The model under review builds one solid part; all positions refer to its coordinate system, in mm. A direction names the side the tool comes from. Round coordinates to 2 decimals unless told otherwise and drop trailing zeros. Loops run counter-clockwise (first coordinate to the right, second up) from the corner with the lowest first, then second, coordinate; pieces in that order, holes last. Notation, with made-up numbers: M 80.5,-28 L 85.5,-28 A18 ccw 85.5,-15 Z; hole C 70,-15.75 d8. An arc over 180 degrees is marked long. Use a Markdown table: item, result. Add a question column.
```python
from build123d import *

# Parameters (mm, degrees)
BOX_W           = 36
BOX_H           = 36
BOX_DEPTH       = 36
SKETCH_R        = 3.5
POCKET_DEPTH    = 36.001
SKETCH004_R     = 7
POCKET001_DEPTH = 13
SKETCH001_R     = 7
POCKET002_DEPTH = 13
SKETCH003_R     = 13
POCKET003_DEPTH = 36.001
SKETCH002_R     = 13
POCKET004_DEPTH = 36.001


with BuildPart() as part:
    # Box → Box (new body)
    with BuildSketch(Plane.XY):
        with Locations((18, 18)):
            Rectangle(BOX_W, BOX_H)
    extrude(amount=BOX_DEPTH)

    # Sketch → Pocket (cut, through all)
    with BuildSketch(Plane.XY.offset(36)):
        with Locations((18, 18)):
            Circle(SKETCH_R)
    extrude(amount=-POCKET_DEPTH, mode=Mode.SUBTRACT)

    # Sketch004 → Pocket001 (cut)
    with BuildSketch(Plane.XY.offset(36)):
        with Locations((18, 18)):
            Circle(SKETCH004_R)
    extrude(amount=-POCKET001_DEPTH, mode=Mode.SUBTRACT)

    # Sketch001 → Pocket002 (cut)
    with BuildSketch(Plane(origin=(0, 0, 0), x_dir=(1, 0, 0), z_dir=(0, 0, -1))):
        with Locations((18, -18)):
            Circle(SKETCH001_R)
    extrude(amount=-POCKET002_DEPTH, mode=Mode.SUBTRACT)

    # Sketch003 → Pocket003 (cut, through all)
    with BuildSketch(Plane(origin=(0, 0, 0), x_dir=(0, -1, 0), z_dir=(-1, 0, 0))):
        with Locations((-18, 36)):
            Circle(SKETCH003_R)
    extrude(amount=-POCKET003_DEPTH, mode=Mode.SUBTRACT)

    # Sketch002 → Pocket004 (cut, through all)
    with BuildSketch(Plane.XZ):
        with Locations((18, 0)):
            Circle(SKETCH002_R)
    extrude(amount=-POCKET004_DEPTH, mode=Mode.SUBTRACT)


solid = part.part
```
(1) For faces 1 (the face through (21, 15, 23)), 2 (the face through (26.573, 17.748, 9.772)), 3 (the face through (25, 18, 12)), list the 3-axis set-ups (+Z, -Z, +X, -X, +Y, -Y) from which the entire face can be reached by the end or side of a thin tool; tool diameter is ignored.
(2) Consider section C-C, the plane x = 21. Give the boundary of the cut face in (y, z).
(3) Insertion check: pin 1 Ø11 at (x, y) = (18, 18) entering from +Z; pin 2 Ø4 at (x, y) = (14.5, 16.5) entering from -Z; pin 3 Ø4 at (x, y) = (18.5, 10) entering from -Z; pin 4 Ø5 at (x, z) = (21.5, 8.5) entering from +Y. Each pin has a flat end and moves straight along its axis. Give the tip position at first contact, or say it passes through.
(4) Consider section D-D, the plane z = 21.5. Give the boundary of the cut face in (x, y).
(5) To check wall thickness, follow probe 1 along Y at (x, z) = (18, 18); probe 2 along Y at (x, z) = (32.5, 24). State the ranges of each line that lie inside material, in increasing order.
(6) Consider section B-B, the plane z = 5.5. Give the boundary of the cut face in (x, y).
Found:
| question | item | result |
|---|---|---|
| 1 | face 1 | +Z |
| 1 | face 2 | -Z, +Y, -Y |
| 1 | face 3 | -Z |
| 2 | outline | M 0,12.65 L 11.68,12.65 L 11.68,13 L 16.2,13 L 16.2,23 L 11.68,23 L 11.68,24.64 A13 cw 5,36 L 0,36 Z; M 19.8,13 L 24.32,13 L 24.32,12.65 L 36,12.65 L 36,36 L 31,36 A13 cw 24.32,24.64 L 24.32,23 L 19.8,23 Z |
| 3 | pin 1 | stops at z = 23 |
| 3 | pin 2 | stops at z = 13 |
| 3 | pin 3 | stops at z = 12.76 |
| 3 | pin 4 | passes through |
| 4 | outline | M 0,0 L 36,0 L 36,36 L 0,36 Z; hole C 18,18 d7 |
| 5 | probe 1 | y = 0 to 14.5, 21.5 to 36 |
| 5 | probe 2 | y = 0 to 13, 23 to 36 |
| 6 | outline | M 0,0 L 6.22,0 L 6.22,36 L 0,36 Z; M 29.78,0 L 36,0 L 36,36 L 29.78,36 Z |
